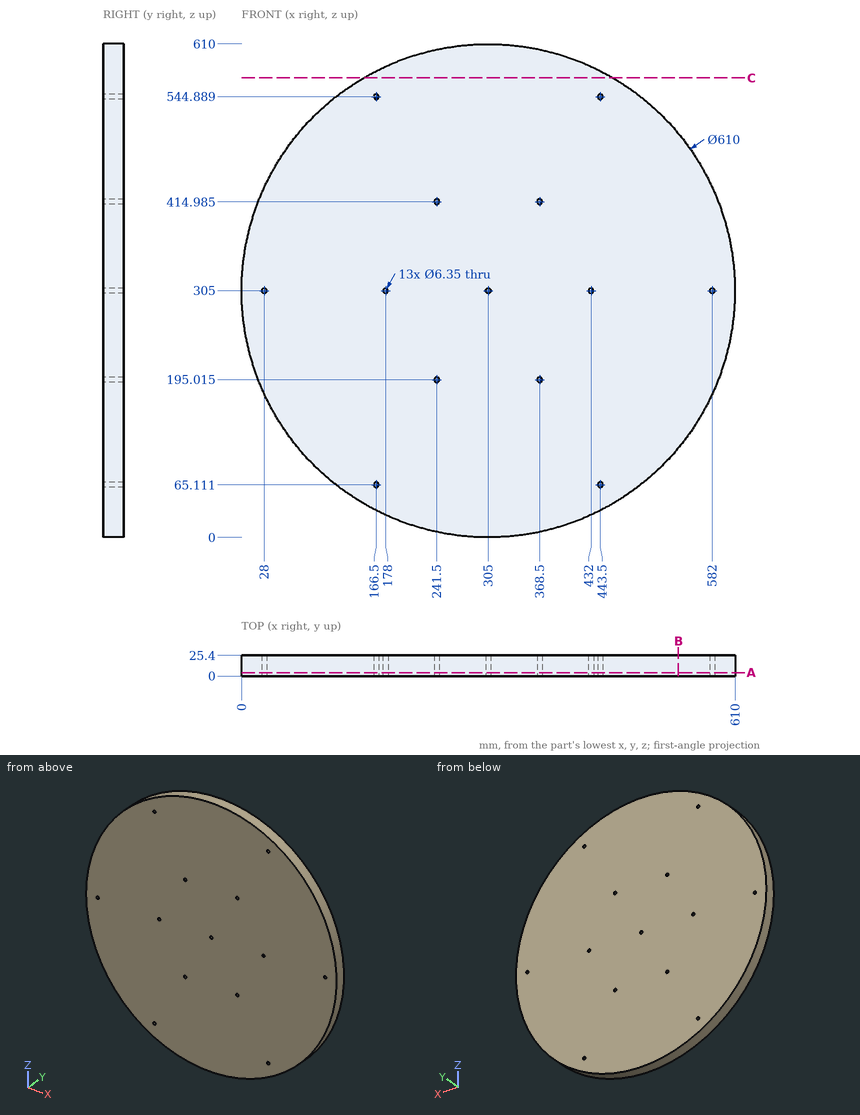
Input: dimensioned drawing with shaded views. Units: mm. Origin: part minimum x, y, z. Give positions to 0.01 mm unless a question says otherwise; leave off trailing zeros. Loops run counter-clockwise (first coordinate to the right, second up) from the corner with the lowest first, then second, coordinate; pieces in that order, holes last. Notation, with made-up numbers: (-4, -13.5) -> (33, -13.5) arc R12 cw to (33, 8.5) -> close; hole circle Ø4 at (65, 52). An arc over 180 degrees is marked (long way). Return JSON: item names as keys, results as strings.
Item 1: Section A-A, the plane y = 4.25. Count the separate pieces of the cut face and the enclosed holes in it, plus the area to 3 significant figures.
Filled in:
{"separate pieces": "1", "enclosed holes": "13", "area": "292,000 mm^2"}
Item 2: Line query: line 1 (Z direction, x = 305, y = 15.75) (3 decimals); line 2 (Z direction, x = 298.5, y = 20.25); line 3 (X direction, y = 8.5, z = 154). Output: solid intervals per line, ascending.
Filled in:
{"line 1": "0 to 301.825, 308.175 to 610", "line 2": "0.07 to 609.93", "line 3": "40 to 570"}
Item 3: Pin query (flat end, axial travel): P1, Ø6, axis at x = 421, y = 20.5, coming from the -Z side (1 decimal); P2, Ø7.5, axis at x = 28, z = 305, coming from the +Y side; P3, Ø1.5, axis at y = 21, z = 73.5, coming from the -X side; P4, Ø5, axis at x = 432, z = 305, coming from the -Y side. Return the tip coordinate at first contact, or that it passes through.
Filled in:
{"P1": "z = 21.7", "P2": "y = 25.4", "P3": "x = 105.55", "P4": "through"}
Item 4: Section C-C, the plane z = 568. Output: boundary loops of the cut face in (x, y).
Filled in:
{"outline": "(150.55, 0) -> (459.45, 0) -> (459.45, 25.4) -> (150.55, 25.4) -> close"}
Item 5: Section B-B, the plane x = 540. Output: boundary loops of the cut face in (y, z).
Filled in:
{"outline": "(0, 110.58) -> (25.4, 110.58) -> (25.4, 499.42) -> (0, 499.42) -> close"}
